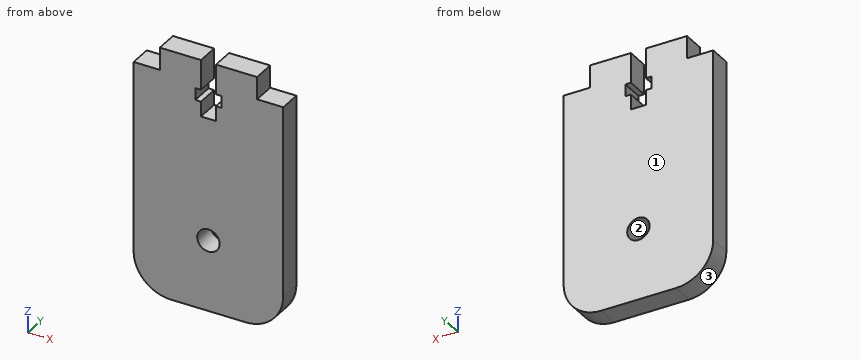
from build123d import *

# Parameters (mm, degrees)
SKETCH1_R           = 3
BOSS_EXTRUDE2_DEPTH = 6


with BuildPart() as part:
    # Sketch1 → Boss-Extrude2 (new body)
    with BuildSketch(Plane(origin=(0, 0, 0), x_dir=(1, 0, 0), z_dir=(0, 1, 0))):
        with BuildLine():
            Line((-10.520184167, 63), (9.479815833, 63))
            ThreePointArc((9.479815833, 63), (16.550883645, 60.071067812), (19.479815833, 53))
            Line((19.479815833, 53), (19.479815833, 2))
            Line((19.479815833, 2), (12.479815833, 2))
            Line((12.479815833, 2), (12.479815833, -4))
            Line((12.479815833, -4), (1.479815833, -4))
            Line((1.479815833, -4), (1.479815833, 4))
            Line((1.479815833, 4), (2.979815833, 4))
            Line((2.979815833, 4), (2.979815833, 7.2))
            Line((2.979815833, 7.2), (1.479815833, 7.2))
            Line((1.479815833, 7.2), (1.479815833, 11.2))
            Line((1.479815833, 11.2), (-2.520184167, 11.2))
            Line((-2.520184167, 11.2), (-2.520184167, 7.2))
            Line((-2.520184167, 7.2), (-4.020184167, 7.2))
            Line((-4.020184167, 7.2), (-4.020184167, 4))
            Line((-4.020184167, 4), (-2.520184167, 4))
            Line((-2.520184167, 4), (-2.520184167, -4))
            Line((-2.520184167, -4), (-13.520184167, -4))
            Line((-13.520184167, -4), (-13.520184167, 2))
            Line((-13.520184167, 2), (-20.520184167, 2))
            Line((-20.520184167, 2), (-20.520184167, 53))
            ThreePointArc((-20.520184167, 53), (-17.591251979, 60.071067812), (-10.520184167, 63))
        make_face()
        with Locations((-0.520184167, 44)):
            Circle(SKETCH1_R, mode=Mode.SUBTRACT)
    extrude(amount=-BOSS_EXTRUDE2_DEPTH)


solid = part.part
Here's how the part is built. I have some questions about the finished solid (model axes, mm). Face numbers are marked on the shaded views. Coordinates: 2 decimals unless noted, no trailing zeros. Write each loop counter-clockwise with the first axis right and the second up, starting at its lowest first coordinate (ties: lowest second). Pieces come first, ordered by that corner, then holes.
Item 1: Will these pins go through, and if not, where does the flat tip stop? pin 1 (3 mm diameter, centred on x = 15.5, y = -2, fed in from +Z); pin 2 (1.8 mm diameter, centred on y = -2.5, z = 0, fed in from -X); pin 3 (3 mm diameter, centred on x = -0.5, y = -4, fed in from +Z).
Item 2: I want a section at B-B on y = -2.6. Write out the boundary of the cut face in (x, z), and give its area (3 significant figures).
Item 3: I want a section at C-C on x = 15. Write out the boundary of the cut face in (y, z).
Item 4: If we mould it in two halves opening along Z, with no side actions, what happens to the marked faces 1, 2 and 3? For each: +Z half, -Z half, draft (parallel to the pull), parting line (faces both ways), or undercut.
Item 5: I want a section at A-A on z = -44. Write out the boundary of the cut face in (x, y).
Item 6: If I drill on line 1 (X direction, y = -2.2, z = -44); line 2 (X direction, y = -5.6, z = -8); line 3 (Z direction, x = -2, y = -4.7), over which ranges is the centre line in solid material (lowest first)?
Findings below:
1. pin 1: stops at z = -2
1. pin 2: stops at x = -13.52
1. pin 3: stops at z = -11.2
2. outline: (-20.52, -53) arc R10 ccw to (-10.52, -63) - (9.48, -63) arc R10 ccw to (19.48, -53) - (19.48, -2) - (12.48, -2) - (12.48, 4) - (1.48, 4) - (1.48, -4) - (2.98, -4) - (2.98, -7.2) - (1.48, -7.2) - (1.48, -11.2) - (-2.52, -11.2) - (-2.52, -7.2) - (-4.02, -7.2) - (-4.02, -4) - (-2.52, -4) - (-2.52, 4) - (-13.52, 4) - (-13.52, -2) - (-20.52, -2) - close; hole circle Ø6 at (-0.52, -44)
2. area: 2,450 mm2
3. outline: (-6, -61.34) - (0, -61.34) - (0, -2) - (-6, -2) - close
4. face 1: draft
4. face 2: undercut
4. face 3: -Z half
5. outline: (-20.52, -6) - (-3.52, -6) - (-3.52, 0) - (-20.52, 0) - close; (2.48, -6) - (19.48, -6) - (19.48, 0) - (2.48, 0) - close
6. line 1: x = -20.52 to -3.52, 2.48 to 19.48
6. line 2: x = -20.52 to -2.52, 1.48 to 19.48
6. line 3: z = -63 to -46.61, -41.39 to -11.2
